from build123d import *

# Parameters (mm, degrees)
SKETCH1_W               = 20.5
SKETCH1_H               = 20.5
BOSS_EXTRUDE1_DEPTH     = 75
SKETCH2_W               = 20.5
SKETCH2_H               = 20.5
SKETCH2_R               = 2.75
BOSS_EXTRUDE2_DEPTH     = 35
CUT_EXTRUDE1_DEPTH      = 26
CUT_EXTRUDE1_DEPTH_BACK = 26


with BuildPart() as part:
    # Sketch1 → Boss-Extrude1 (new body)
    with BuildSketch(Plane.XY):
        Polygon((-25, -35), (-14.832007533, 12.739060279), (-12.321067812, 15.25), (12.321067812, 15.25), (14.832007533, 12.739060279), (25, -35), align=None)
        Rectangle(SKETCH1_W, SKETCH1_H, mode=Mode.SUBTRACT)
    extrude(amount=BOSS_EXTRUDE1_DEPTH)

    # Sketch2 → Boss-Extrude2 (add)
    with BuildSketch(Plane.XY.offset(75)):
        Rectangle(SKETCH2_W, SKETCH2_H)
        Circle(SKETCH2_R, mode=Mode.SUBTRACT)
    extrude(amount=-BOSS_EXTRUDE2_DEPTH)

    # Sketch3 → Cut-Extrude1 (cut, two sides)
    with BuildSketch(Plane(origin=(0, 0, 0), x_dir=(0, 0, -1), z_dir=(1, 0, 0))) as cut_extrude1_sk:
        Polygon((0, -15.25), (-28.597332184, -15.25), (-40, -35), (0, -35), align=None)
        Polygon((-45, 15.25), (-75, -36.711524227), (-75, 15.25), align=None)
    extrude(amount=CUT_EXTRUDE1_DEPTH, mode=Mode.SUBTRACT)
    extrude(cut_extrude1_sk.sketch, amount=-CUT_EXTRUDE1_DEPTH_BACK, mode=Mode.SUBTRACT)


solid = part.part
For this review, take the finished solid that the model builds, in its own axes (mm). A direction names the side the tool comes from. Give positions to 0.01 mm unless a question says otherwise; leave off trailing zeros. Order: outer loops, then holes, each group sorted by start corner. A loop starts at its lowest first (then second) coordinate and runs counter-clockwise, first axis right, second up. Notation, with made-up numbers: M 65,12 L 113,12 A25 ccw 113,48 Z; hole C 15.5,83 d5. An arc over 180 degrees is marked long. Answer in a Markdown table with one row per item. Add a question column.
(1) Wall thickness on probe 1 along Y at (x, z) = (-6, 7); probe 2 along Y at (x, z) = (0, 45); probe 3 along X at (y, z) = (5.5, 13.5): over which ranges is each line inside the solid? List them lowest first. Write a range as [from, to].
(2) Consider section A-A on z = 16. State the section outline as (x, y) points.
(3) For faces 1 (the face through (0, -15.25, 14)), 2 (the face through (-19.987, -11.465, 36.488)), 3 (the face through (0, -10.25, 20)), list the 3-axis set-ups (+Z, -Z, +X, -X, +Y, -Y) from which the entire face can be reached by the end or side of a thin tool; tool diameter is ignored.
(4) Consider section C-C on y = -9. State the section outline as (x, z) points.
(5) Mouldability with a two-part tool opening along Y and no side actions: class faces 4 (the face through (13.56, 14.01, 22.9)), 5 (the face through (0.35, -24.99, 34.22)), 6 (the face through (0, 10.25, 20)) as +Y half, -Y half, draft (parallel to the pull), parting line (faces both ways), or undercut.
(6) For pin 1 (4 mm diameter, centred on x = 8, y = -15.5, fed in from +Z); pin 2 (1 mm diameter, centred on x = 0.5, y = -7, fed in from -Z); pin 3 (16.5 mm diameter, centred on x = 0.5, z = 26.5, fed in from -Y); pin 4 (4.5 mm diameter, centred on x = 0, y = 0, fed in from -Z), all flat-tipped, find the tip position at first contact; note any pin that passes through.
(7) Consider section D-D on z = 34. State the section outline as (x, y) points.
(8) Consider section B-B on x = -6.5. State the section outline as (y, z) points, and give its area (3 significant figures).
Evaluation:
| question | item | result |
|---|---|---|
| 1 | probe 1 | y = [-15.25, -10.25], [10.25, 15.25] |
| 1 | probe 2 | y = [-35, -2.75], [2.75, 15.25] |
| 1 | probe 3 | x = [-16.37, -10.25], [10.25, 16.37] |
| 2 | outline | M -20.79,-15.25 L 20.79,-15.25 L 14.83,12.74 L 12.32,15.25 L -12.32,15.25 L -14.83,12.74 Z; hole M -10.25,-10.25 L 10.25,-10.25 L 10.25,10.25 L -10.25,10.25 Z |
| 3 | face 1 | -Z, +X, -X, -Y |
| 3 | face 2 | +Z, -Z, -X, +Y |
| 3 | face 3 | -Z |
| 4 | outline | M -19.46,0 L -10.25,0 L -10.25,40 L 10.25,40 L 10.25,0 L 19.46,0 L 19.46,59 L -19.46,59 Z |
| 5 | face 4 | +Y half |
| 5 | face 5 | -Y half |
| 5 | face 6 | undercut |
| 6 | pin 1 | stops at z = 63.91 |
| 6 | pin 2 | stops at z = 40 |
| 6 | pin 3 | stops at y = -25.91 |
| 6 | pin 4 | passes through |
| 7 | outline | M -22.79,-24.61 L 22.79,-24.61 L 14.83,12.74 L 12.32,15.25 L -12.32,15.25 L -14.83,12.74 Z; hole M -10.25,-10.25 L 10.25,-10.25 L 10.25,10.25 L -10.25,10.25 Z |
| 8 | outline | M -35,40 L -15.25,28.6 L -15.25,0 L -10.25,0 L -10.25,40 L 10.25,40 L 10.25,0 L 15.25,0 L 15.25,45 L -35,74.01 Z |
| 8 | area | 1,490 mm^2 |
